Source: CAD feature listing. Evaluate the final solid. Frame: model axes, mm. Face numbers are marked on the shaded views. A direction names the side the tool comes from. Round coordinates to 2 decimals unless told otherwise and drop trailing zeros. Write each loop counter-clockwise with the first axis right and the second up, starting at its lowest first coordinate (ties: lowest second). Pieces come first, ordered by that corner, then holes.
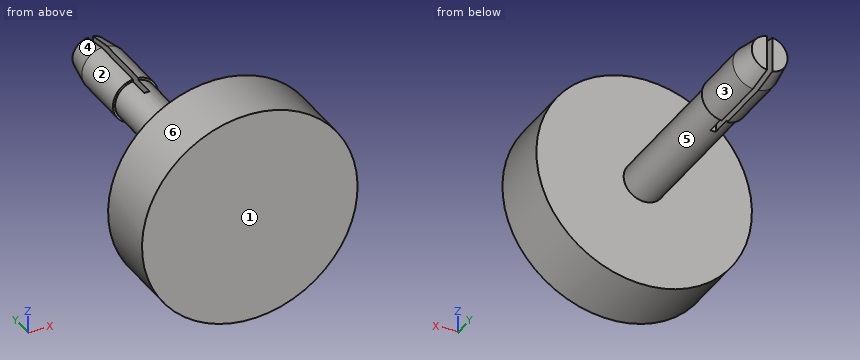
from build123d import *

# Parameters (mm, degrees)
ESQUISSE2_R             = 5
BOSS_EXTRU_1_DEPTH      = 3
ESQUISSE3_R             = 0.95
BOSS_EXTRU_2_DEPTH      = 7.1
ESQUISSE4_R             = 1.05
BOSS_EXTRU_3_DEPTH      = 4
CHANFREIN3_SIZE         = 1.25
CHANFREIN3_SIZE2        = 0.220408726
ESQUISSE5_W             = 0.25
ESQUISSE5_H             = 3
ENL_V_MAT_EXTRU_1_DEPTH = 5


with BuildPart() as part:
    # Esquisse2 → Boss.-Extru.1 (new body)
    with BuildSketch(Plane(origin=(0, 0, 0), x_dir=(1, 0, 0), z_dir=(0, 1, 0))):
        with Locations(Location((0, 0, 0), (0, 0, 270))):
            Circle(ESQUISSE2_R)
    extrude(amount=BOSS_EXTRU_1_DEPTH)

    # Esquisse3 → Boss.-Extru.2 (add)
    with BuildSketch(Plane(origin=(0, 3, 0), x_dir=(1, 0, 0), z_dir=(0, 1, 0))):
        with Locations(Location((0, 0, 0), (0, 0, 270))):
            Circle(ESQUISSE3_R)
    extrude(amount=BOSS_EXTRU_2_DEPTH)

    # Esquisse4 → Boss.-Extru.3 (add)
    with BuildSketch(Plane(origin=(0, 10.1, 0), x_dir=(1, 0, 0), z_dir=(0, 1, 0))):
        with Locations(Location((0, 0, 0), (0, 0, 270))):
            Circle(ESQUISSE4_R)
    extrude(amount=BOSS_EXTRU_3_DEPTH)

    # Chanfrein3
    chanfrein3_edges = [part.edges().sort_by_distance(p)[0] for p in [
        (0, 14.1, -1.05),
    ]]
    chanfrein3_side = [part.faces().sort_by_distance(p)[0] for p in [
        (0, 12.1, -1.05),
    ]]
    chamfer(chanfrein3_edges, length=CHANFREIN3_SIZE, length2=CHANFREIN3_SIZE2, reference=chanfrein3_side[0])

    # Esquisse5 → Enlèv. mat.-Extru.1 (cut)
    with BuildSketch(Plane(origin=(0, 14.1, 0), x_dir=(1, 0, 0), z_dir=(0, 1, 0))):
        Rectangle(ESQUISSE5_W, ESQUISSE5_H)
    extrude(amount=-ENL_V_MAT_EXTRU_1_DEPTH, mode=Mode.SUBTRACT)


solid = part.part
1) Pull-direction query (Y, two-part tool) for the marked faces 4, 5 and 6; classes: released by +Y, released by -Y, zero draft, split by the parting line, or undercut.
Taken from the geometry:
face 4: released by +Y
face 5: undercut
face 6: zero draft
2) Section query B-B on y = 7.75. Return the cut outline in (x, z).
Taken from the geometry:
outline: circle Ø1.9 at (0, 0)
3) Contact query for flat-ended pins moving along their axis: P1, Ø3, axis at x = -1.5, z = 3.5, coming from the +Y side; P2, Ø1, axis at y = 10.5, z = 0, coming from the +X side; P3, Ø1.7, axis at y = 10.5, z = 0.5, coming from the -X side; P4, Ø1.5, axis at y = 6.5, z = 2, coming from the +X side. Output: stop coordinate, or through.
Taken from the geometry:
P1: stops at y = 3
P2: stops at x = 1.05
P3: stops at x = -1.05
P4: passes through
4) Reachability of the marked faces 1, 2 and 3 from +Z, -Z, +X, -X, +Y, -Y: full face, straight path, thin tool, end or side. Return the list, or none.
Taken from the geometry:
face 1: +Z, -Z, +X, -X, -Y
face 2: -X, +Y
face 3: +X, +Y
5) Section query A-A on z = 0. Return the cut outline in (x, y) (3 decimals).
Taken from the geometry:
outline: (-5, 0) - (5, 0) - (5, 3) - (0.95, 3) - (0.95, 10.1) - (1.05, 10.1) - (1.05, 12.85) - (0.83, 14.1) - (0.125, 14.1) - (0.125, 9.1) - (-0.125, 9.1) - (-0.125, 14.1) - (-0.83, 14.1) - (-1.05, 12.85) - (-1.05, 10.1) - (-0.95, 10.1) - (-0.95, 3) - (-5, 3) - close
6) Material intervals for line 1 (Y direction, x = 0.5, z = -3.25); line 2 (X direction, y = 9.5, z = -0.75) (3 decimals); line 3 (X direction, y = 2, z = 4.25), sorted ascending.
Taken from the geometry:
line 1: y = 0 to 3
line 2: x = -0.583 to -0.125, 0.125 to 0.583
line 3: x = -2.63 to 2.63
7) Section query D-D on z = 4. Return the cut outline in (x, y), then the cut area to 3 significant figures.
Taken from the geometry:
outline: (-3, 0) - (3, 0) - (3, 3) - (-3, 3) - close
area: 18.0 mm2
8) Section query C-C on x = -4. Return the cut outline in (y, z).
Taken from the geometry:
outline: (0, -3) - (3, -3) - (3, 3) - (0, 3) - close
